Answer from the drawing. Dimensions are ordinates in mm from the lowest x, y and z of the part. Give positions to 0.01 mm unless a question says otherwise; leave off trailing zeros. Order: outer loops, then holes, each group sorted by start corner. A loop starts at its lowest first (then second) coordinate and runs counter-clockwise, first axis right, second up. Notation, with made-up numbers: (-37, 0.25) - (-32, 0.25) arc R31 ccw to (-32, 37.25) - close; hole circle Ø10 at (65.25, 51.25). An arc over 180 degrees is marked (long way). Write each question's results on one line, items separated by ' | '.
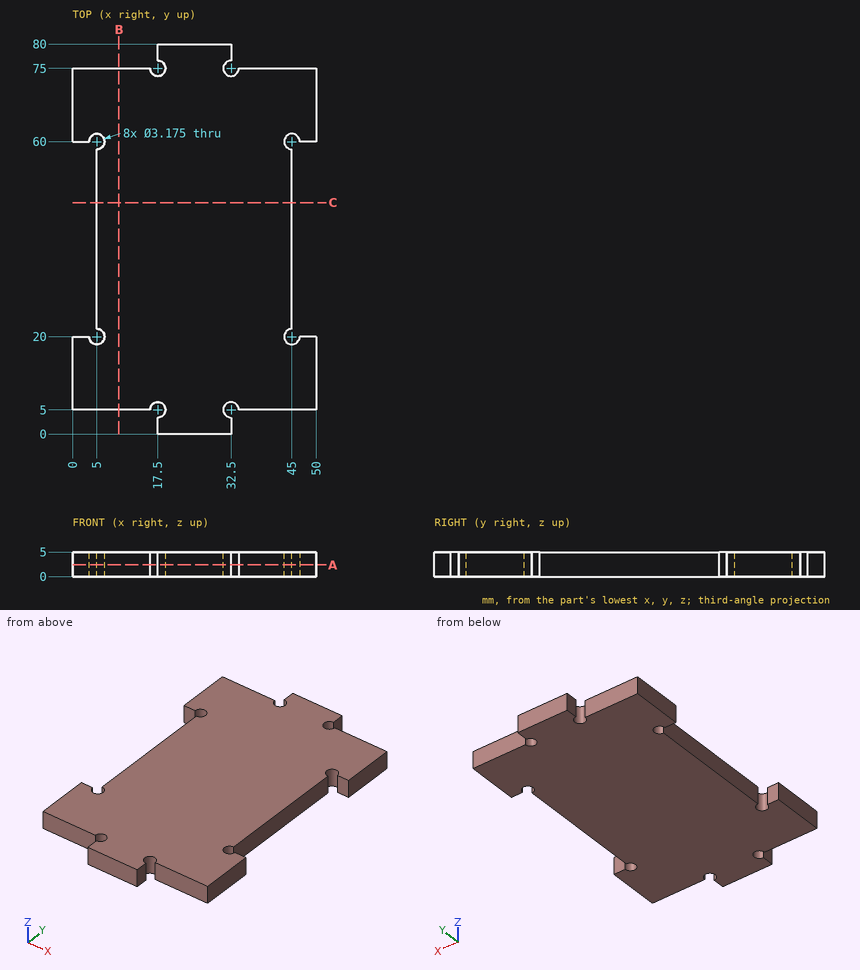
(1) Consider probe 1 along X at (y, z) = (57.5, 1.45); probe 2 along Y at (x, z) = (10.5, 3.65); probe 3 along Y at (x, z) = (4.5, 3.6). Determine where each line is inside the solid, lowest interval first. Write a range as [from, to].
Conclusion:
probe 1: [5, 45] | probe 2: [5, 75] | probe 3: [5, 18.49], [61.51, 75]
(2) Section A-A (z = 2.4) is taken. Give the vertices of the cut face in (x, y) (1 decimal), plus the area to 3 significant figures.
Conclusion:
outline: (0, 5) - (15.9, 5) arc R1.6 cw (long way) to (17.5, 3.4) - (17.5, 0) - (32.5, 0) - (32.5, 3.4) arc R1.6 cw (long way) to (34.1, 5) - (50, 5) - (50, 20) - (46.6, 20) arc R1.6 cw (long way) to (45, 21.6) - (45, 58.4) arc R1.6 cw (long way) to (46.6, 60) - (50, 60) - (50, 75) - (34.1, 75) arc R1.6 cw (long way) to (32.5, 76.6) - (32.5, 80) - (17.5, 80) - (17.5, 76.6) arc R1.6 cw (long way) to (15.9, 75) - (0, 75) - (0, 60) - (3.4, 60) arc R1.6 cw (long way) to (5, 58.4) - (5, 21.6) arc R1.6 cw (long way) to (3.4, 20) - (0, 20) - close | area: 3,200 mm^2
(3) Each of these flat-tipped pins is pushed along its axis until it touches: pin 1 (2 mm diameter, centred on x = 8.5, y = 59, fed in from -Z); pin 2 (2.5 mm diameter, centred on x = 49, z = 2.5, fed in from -Y); pin 3 (2.5 mm diameter, centred on y = 1, z = 2.5, fed in from -X); pin 4 (2.5 mm diameter, centred on y = 47.5, z = 2, fed in from -X). Where does it stop, or does it pass through?
Conclusion:
pin 1: z = 0 | pin 2: y = 5 | pin 3: x = 17.5 | pin 4: x = 5
(4) Section B-B (x = 9.5) is taken. Give the vertices of the cut face in (y, z), plus the area to 3 significant figures.
Conclusion:
outline: (5, 0) - (75, 0) - (75, 5) - (5, 5) - close | area: 350 mm^2
(5) Section C-C (y = 47.5) is taken. Give the vertices of the cut face in (x, z).
Conclusion:
outline: (5, 0) - (45, 0) - (45, 5) - (5, 5) - close
